Input: part model. Units: mm. Frame: model coordinates. A direction names the side the tool comes from. Coordinates: 2 decimals unless noted, no trailing zeros. Order: outer loops, then holes, each group sorted by start corner. A loop starts at its lowest first (then second) coordinate and runs counter-clockwise, first axis right, second up. Notation, with made-up numbers: (-38, 12.25) - (-20, 12.25) arc R27 cw to (-20, 32.25) - close; hole circle Ø2 at (55.25, 81.25). An arc over 180 degrees is marked (long way). One line per question, with ' | ' between items. Start each with the question number.
```python
from build123d import *

# Parameters (mm, degrees)
BOSS_EXTRU_1_DEPTH = 120
CONG_1_R           = 2
CONG_2_R           = 2
COQUE1_DEPTH       = 117


# Read off the part's stored shape, not the designer's step: Coque1
with BuildPart() as part:
    # Esquisse2 → Boss.-Extru.1 (new body)
    with BuildSketch(Plane.XY):
        with BuildLine():
            ThreePointArc((84.733796148, 26.7419608), (0, 37.829829119), (-84.733796148, 26.7419608))
            ThreePointArc((-84.733796148, 26.7419608), (-111.556110074, -19.547945422), (-65.266203852, -46.370259347))
            ThreePointArc((-65.266203852, -46.370259347), (0, -37.829829119), (65.266203852, -46.370259347))
            ThreePointArc((65.266203852, -46.370259347), (111.556110074, -19.547945422), (84.733796148, 26.7419608))
        make_face()
    extrude(amount=BOSS_EXTRU_1_DEPTH)

    # Congé1
    cong_1_edges = [part.edges().sort_by_distance(p)[0] for p in [
        (-111.556110074, -19.547945422, 120),
        (0, -37.829829119, 120),
        (111.556110074, -19.547945422, 120),
        (0, 37.829829119, 120),
    ]]
    fillet(cong_1_edges, radius=CONG_1_R)

    # Congé2
    cong_2_edges = [part.edges().sort_by_distance(p)[0] for p in [
        (0, -37.829829119, 0),
        (-111.556110074, -19.547945422, 0),
        (0, 37.829829119, 0),
        (111.556110074, -19.547945422, 0),
    ]]
    fillet(cong_2_edges, radius=CONG_2_R)

    # Coque1 outline → Coque1 (cut)
    with BuildSketch(Plane.XY):
        with BuildLine():
            ThreePointArc((66.038118215, -43.471268451), (108.657119178, -18.776031059), (83.961881785, 23.842969904))
            ThreePointArc((83.961881785, 23.842969904), (0, 34.829829119), (-83.961881785, 23.842969904))
            ThreePointArc((-83.961881785, 23.842969904), (-108.657119178, -18.776031059), (-66.038118215, -43.471268451))
            ThreePointArc((-66.038118215, -43.471268451), (0, -34.829829119), (66.038118215, -43.471268451))
        make_face()
    extrude(amount=COQUE1_DEPTH, mode=Mode.SUBTRACT)


solid = part.part
```
(1) Reachability of faces 1 (the face through (16, 35, 0)), 2 (the face through (-108.846, -18.034, 57.681)) from +Z, -Z, +X, -X, +Y, -Y: full face, straight path, thin tool, end or side. Return the list, or none.
(2) Section A-A (z = 29.5). Output: boundary loops of the cut face in (x, y), then the cut area to 3 significant figures.
(3) Material intervals for line 1 along X through (y, z) = (-18, 94); line 2 along Y through (x, z) = (-77.5, 33); line 3 along Y through (x, z) = (-83, 90), sorted ascending. Write a range as from..to.
(4) Draft query along Y for faces 3 (the face through (1.2, 37.828, 59.188)), 4 (the face through (-111.76, -18.74, 59.19)), 5 (the face through (-2, -4, 117)), 6 (the face through (-2, -4, 120)). Return one class per face: +Y half, -Y half, draft (parallel to the pull), parting line (faces both ways), or undercut.
(5) Pin query (flat end, axial travel): pin 1 (4 mm diameter, centred on x = 85.5, y = 0, fed in from -Z); pin 2 (2 mm diameter, centred on y = -5.5, z = 68.5, fed in from +X); pin 3 (3 mm diameter, centred on y = 0.5, z = 65, fed in from +X). Return the tip coordinate at first contact, or that it passes through.
Worked answers:
1) face 1: -Z, +X, -X, +Y, -Y | face 2: -Z
2) outline: (-84.73, 26.74) arc R37.83 ccw to (-65.27, -46.37) arc R253.65 cw to (65.27, -46.37) arc R37.83 ccw to (84.73, 26.74) arc R329.31 ccw to start; hole (-83.96, 23.84) arc R34.83 ccw to (-66.04, -43.47) arc R256.65 cw to (66.04, -43.47) arc R34.83 ccw to (83.96, 23.84) arc R326.31 ccw to start | area: 1,600 mm²
3) line 1: x = -111.93..-108.85, 108.85..111.93 | line 2: y = -47.56..-44.55, 25.49..28.58 | line 3: y = -46.79..-43.71, 24.1..27.2
4) face 3: +Y half | face 4: parting line | face 5: undercut | face 6: draft
5) pin 1: stops at z = 117 | pin 2: stops at x = 112.68 | pin 3: stops at x = 111.79
